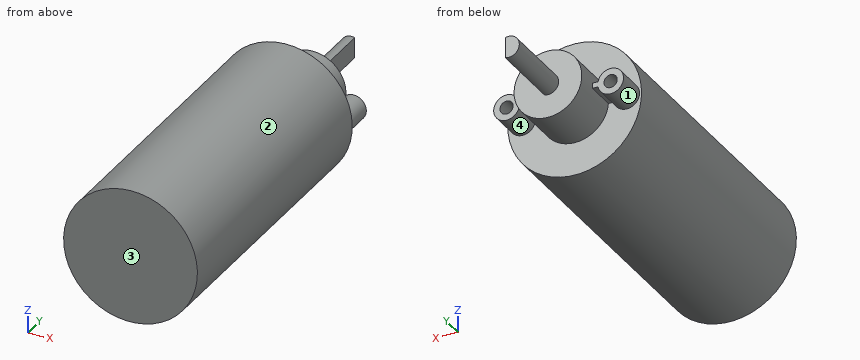
```python
from build123d import *

# Parameters (mm, degrees)
SKETCH1_R           = 10.287
BOSS_EXTRUDE1_DEPTH = 45.974
SKETCH2_R           = 5.207
BOSS_EXTRUDE2_DEPTH = 7.9375
SKETCH3_R           = 1.651
BOSS_EXTRUDE3_DEPTH = 11.684
SKETCH4_R           = 1.984375
SKETCH4_R_2         = 1.016
SKETCH4_W           = 12.957418184
SKETCH4_H           = 0.81
BOSS_EXTRUDE5_DEPTH = 4.7625
CUT_EXTRUDE1_DEPTH  = 11.684


with BuildPart() as part:
    # Sketch1 → Boss-Extrude1 (new body)
    with BuildSketch(Plane(origin=(0, 0, 0), x_dir=(1, 0, 0), z_dir=(0, 1, 0))):
        with Locations(Location((0, 0, 0), (0, 0, 270))):
            Circle(SKETCH1_R)
    extrude(amount=BOSS_EXTRUDE1_DEPTH)

    # Sketch2 → Boss-Extrude2 (add)
    with BuildSketch(Plane(origin=(0, 45.974, 0), x_dir=(1, 0, 0), z_dir=(0, 1, 0))):
        with Locations(Location((0, 0, 0), (0, 0, 270))):
            Circle(SKETCH2_R)
    extrude(amount=BOSS_EXTRUDE2_DEPTH)

    # Sketch3 → Boss-Extrude3 (add)
    with BuildSketch(Plane(origin=(0, 53.9115, 0), x_dir=(1, 0, 0), z_dir=(0, 1, 0))):
        with Locations(Location((0, 0, 0), (0, 0, 270))):
            Circle(SKETCH3_R)
    extrude(amount=BOSS_EXTRUDE3_DEPTH)

    # Sketch4 → Boss-Extrude5 (add)
    # profile 1 of 3: a face of its own
    with BuildSketch(Plane(origin=(0, 45.974, 0), x_dir=(1, 0, 0), z_dir=(0, 1, 0))):
        with Locations((-8.001, 0)):
            Circle(SKETCH4_R)
        with Locations(Location((-8.001, 0, 0), (0, 0, 90))):
            Circle(SKETCH4_R_2, mode=Mode.SUBTRACT)
    # profile 2 of 3: a face of its own
    with BuildSketch(Plane(origin=(0, 45.974, 0), x_dir=(1, 0, 0), z_dir=(0, 1, 0))):
        with Locations((8.001, 0)):
            Circle(SKETCH4_R)
        with Locations(Location((8.001, 0, 0), (0, 0, 90))):
            Circle(SKETCH4_R_2, mode=Mode.SUBTRACT)
    # profile 3 of 3: a face of its own
    with BuildSketch(Plane(origin=(0, 45.974, 0), x_dir=(1, 0, 0), z_dir=(0, 1, 0))):
        with Locations((0.016128597, 0)):
            Rectangle(SKETCH4_W, SKETCH4_H)
    extrude(amount=BOSS_EXTRUDE5_DEPTH)

    # Sketch5 → Cut-Extrude1 (cut)
    with BuildSketch(Plane(origin=(0, 65.5955, 0), x_dir=(1, 0, 0), z_dir=(0, 1, 0))):
        Polygon((0.508, 43.642192231), (0.508, 1.570903243), (0.508, -1.570903243), (0.508, -43.642192231), (84.650577975, -43.642192231), (84.650577975, 43.642192231), align=None)
    extrude(amount=-CUT_EXTRUDE1_DEPTH, mode=Mode.SUBTRACT)


solid = part.part
```
Here's how the part is built. I have some questions about the finished solid (model axes, mm). Face numbers are marked on the shaded views. Coordinates: 2 decimals unless noted, no trailing zeros. Write each loop counter-clockwise with the first axis right and the second up, starting at its lowest first coordinate (ties: lowest second). Pieces come first, ordered by that corner, then holes. Notation, with made-up numbers: (74, 46.25) -> (88, 46.25) arc R9 cw to (88, 57.25) -> close; hole circle Ø8 at (71, 81). An arc over 180 degrees is marked (long way). Use a Markdown table: item, result. Add a question column.
(1) If we section it at A-A, the plane x = -1: Write out the boundary of the cut face in (y, z).
(2) If we section it at C-C, the plane y = 32: Write out the boundary of the cut face in (x, z), and give its area (3 significant figures).
(3) I'm going to push flat-ended pins straight in: P1, Ø3.5, axis at y = 59.5, z = -0.5, coming from the +X side; P2, Ø0.6, axis at x = -8, z = 0, coming from the +Y side; P3, Ø10, axis at y = 39, z = 8, coming from the -X side. Where does each tip first touch, or does it pass through?
(4) If we section it at B-B, the plane z = 3.5: Write out the boundary of the cut face in (x, y).
(5) Please list where these lines run through material, in increasing order: line 1 (X direction, y = 47.7, z = 0) (3 decimals); line 2 (X direction, y = 31, z = 2.5); line 3 (Y direction, x = 1, z = -1.25).
(6) If we section it at D-D, the plane x = 3.25: Write out the boundary of the cut face in (y, z).
(7) We'd pull the mould along X, two halves only. Please class the marked faces 1, 2, 3 and 4: +X half, -X half, draft (parallel to the pull), parting line (faces both ways), or undercut.
Outcome:
| question | item | result |
|---|---|---|
| 1 | outline | (0, -10.24) -> (45.97, -10.24) -> (45.97, -5.11) -> (53.91, -5.11) -> (53.91, -1.31) -> (65.6, -1.31) -> (65.6, 1.31) -> (53.91, 1.31) -> (53.91, 5.11) -> (45.97, 5.11) -> (45.97, 10.24) -> (0, 10.24) -> close |
| 2 | outline | circle Ø20.57 at (0, 0) |
| 2 | area | 332 mm^2 |
| 3 | P1 | stops at x = 0.51 |
| 3 | P2 | stops at y = 45.97 |
| 3 | P3 | stops at x = -9.84 |
| 4 | outline | (-9.67, 0) -> (9.67, 0) -> (9.67, 45.97) -> (3.86, 45.97) -> (3.86, 53.91) -> (-3.86, 53.91) -> (-3.86, 45.97) -> (-9.67, 45.97) -> close |
| 5 | line 1 | x = -9.985 to -9.017, -6.985 to 6.985, 9.017 to 9.985 |
| 5 | line 2 | x = -9.98 to 9.98 |
| 5 | line 3 | y = 0 to 53.91 |
| 6 | outline | (0, -9.76) -> (45.97, -9.76) -> (45.97, -4.07) -> (53.91, -4.07) -> (53.91, 4.07) -> (45.97, 4.07) -> (45.97, 9.76) -> (0, 9.76) -> close |
| 7 | face 1 | undercut |
| 7 | face 2 | parting line |
| 7 | face 3 | draft |
| 7 | face 4 | undercut |
